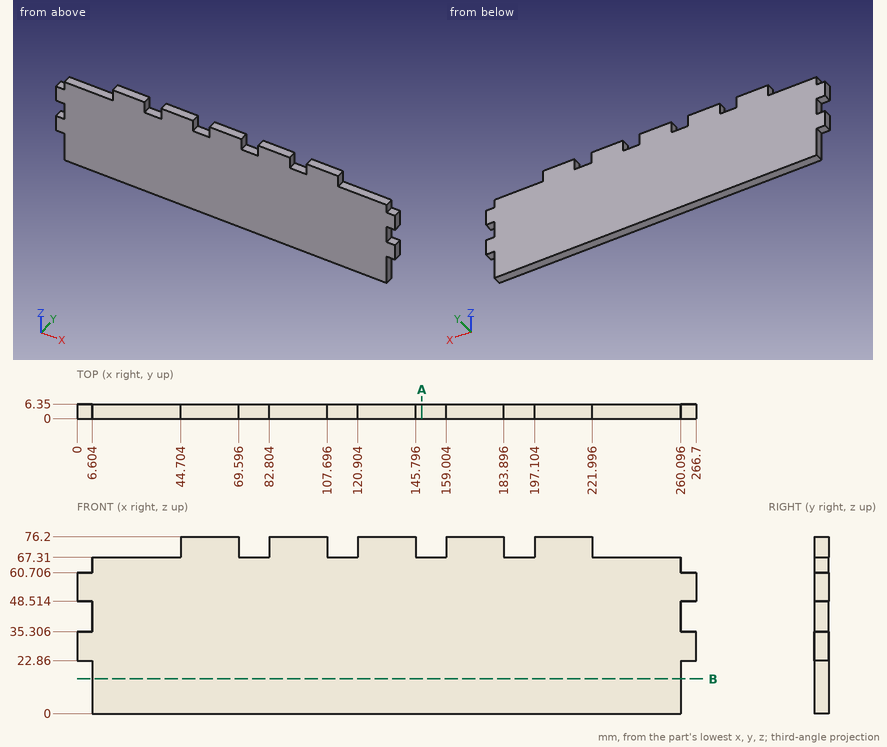
Geometry check sheet. Reference: drawing and pictorial views, mm from the part's lowest x, y, z. Round coordinates to 2 decimals unless told otherwise and drop trailing zeros. Order: outer loops, then holes, each group sorted by start corner. A loop starts at its lowest first (then second) coordinate and runs counter-clockwise, first axis right, second up. Notation, with made-up numbers: (77.5, 65.25) -> (106.5, 65.25) arc R33 ccw to (106.5, 97.25) -> close; hole circle Ø2 at (68.5, 38). An arc over 180 degrees is marked (long way). One line per item, written item: value. Start each with the question number.
Q1. Gauge pin test, flat ends, axial feed: pin 1 Ø5 at (x, z) = (192.5, 37) entering from -Y; pin 2 Ø1.9 at (y, z) = (2, 73.5) entering from +X; pin 3 Ø1.9 at (y, z) = (3.5, 69.5) entering from -X; pin 4 Ø1.9 at (y, z) = (4, 63) entering from +X. Record the tip position at first contact, or that the pin passes through.
Q2. Thickness scan on line 1 (X direction, y = 3.75, z = 68); line 2 (X direction, y = 2, z = 37.5); line 3 (Z direction, x = 19, y = 4.25). Record the ranges inside material, lowest first.
Q3. Cross-section at A-A (x = 148.5). Record the boundary of the cut face in (y, z), and give its area (3 significant figures).
Q4. Cross-section at B-B (z = 15). Record the boundary of the cut face in (x, y).
Completed:
1. pin 1: stops at y = 0
1. pin 2: stops at x = 222
1. pin 3: stops at x = 44.7
1. pin 4: stops at x = 260.1
2. line 1: x = 44.7 to 69.6, 82.8 to 107.7, 120.9 to 145.8, 159 to 183.9, 197.1 to 222
2. line 2: x = 6.6 to 260.1
2. line 3: z = 0 to 67.31
3. outline: (0, 0) -> (6.35, 0) -> (6.35, 67.31) -> (0, 67.31) -> close
3. area: 427 mm²
4. outline: (6.6, 0) -> (260.1, 0) -> (260.1, 6.35) -> (6.6, 6.35) -> close
